Check sheet for the modelled part. Datum: model origin and axes. Units: mm. A direction names the side the tool comes from. Round coordinates to 2 decimals unless told otherwise and drop trailing zeros. Write each loop counter-clockwise with the first axis right and the second up, starting at its lowest first coordinate (ties: lowest second). Pieces come first, ordered by that corner, then holes. Notation, with made-up numbers: (14, -35) -> (37, -35) arc R14 cw to (37, -23) -> close; hole circle Ø10 at (5.5, -19.5). An arc over 180 degrees is marked (long way). Answer as a JSON object with one key per item and string values. Group by question number.
```python
from build123d import *

# Parameters (mm, degrees)
F3_DEPTH        = 70.001
F3_COPIES_COUNT = 20


# Not quite as in the source:
# - a feature of the source that left no trace in its solid (it failed there, or was rolled back) is left out
# - a pattern or mirror of a feature is missing from the dataset's text; its kind, count and spacing are read off the source's solid


with BuildPart() as f1:
    # F0 (on Front) → F1 (revolve)
    with BuildSketch(Plane.XZ):
        Polygon((35, -20), (35, 20), (-35, 20), (-35, -20), (-15, -20), (-15, -37.5), (-35, -37.5), (-35, -62.5), (35, -62.5), (35, -37.5), (15, -37.5), (15, -20), align=None)
    revolve(axis=Axis((-7.5, 0, -80), (-1, 0, 0)))

    # F2 (on face) → F3 (cut, through all)
    with BuildSketch(Plane.YZ.offset(35)):
        with BuildLine():
            ThreePointArc((-2.4875303205, 5.9552673354), (0.9594167449, 5.9859018055), (4.4048221019, 5.878363585))
            ThreePointArc((4.4048221019, 5.878363585), (5.5383005859, 6.1619770528), (6.3198858178, 7.0305014326))
            Line((6.3198858178, 7.0305014326), (12.0290632191, 19.2738718801))
            ThreePointArc((12.0290632191, 19.2738718801), (0, 20), (-12.0290632191, 19.2738718801))
            Line((-12.0290632191, 19.2738718801), (-7.1637078206, 8.8400835574))
            ThreePointArc((-7.1637078206, 8.8400835574), (-5.2573859952, 6.6977976646), (-2.4875303205, 5.9552673354))
        make_face()
    f3 = extrude(amount=-F3_DEPTH, mode=Mode.SUBTRACT)

    # F3_copies: F3 ×20 about axis
    f3_copies_axis = Axis((0, 0, -80), (1, 0, 0))
    for i in range(1, F3_COPIES_COUNT):
        add(f3.rotate(f3_copies_axis, i * 360 / F3_COPIES_COUNT), mode=Mode.SUBTRACT)


solid = f1.part
```
(1) Scan lines: line 1 along Y through (x, z) = (28.25, -80); line 2 along Z through (x, y) = (-27.5, 3); line 3 along Z through (x, y) = (-9.5, -87). Record each from-to range of solid material in increasing order.
(2) Release check for a two-part mould opening along Y. For faces 4 (the flat face through (0.49, 86.55, -41.75)), 5 (the cylindrical face through (0.49, 5.29, -166.72)), 6 (the cylindrical face through (-0.5, -45.4, 9.1)) record: pulls with the +Y half, pulls with the -Y half, needs draft (parallel to the pull), parting line crosses it, or undercut.
(3) Access from +Z, -Z, +X, -X, +Y, -Y to the whole of each face (thin tool, end or side, straight path). Record for faces 1 (the flat face through (0.49, -47.313, 0.661)), 2 (the flat face through (0.49, 69.92, -142.09)), 3 (the flat face through (0.49, -63.119, -9.508)).
(4) Section check C-C on x = 22.5. State how many separate pieces and enclosed holes the cut face has, then the cut area to 3 significant figures.
(5) Section check B-B on y = 0. Record the cut outline in (x, z).
(6) Go/stop test with flat-tipped pins: pin 1 Ø10 at (x, z) = (21, -53.5) entering from -Y; pin 2 Ø1 at (x, y) = (7, -59) entering from +Z; pin 3 Ø2 at (x, z) = (8, -0.5) entering from +Y. Record where each tip stops, or that it passes through.
(7) Section check A-A on z = -80. Record the cut outline in (x, y).
Data:
{
 "1": {"line 1": "y = -85.99 to -60, -42.5 to -17.5, 17.5 to 42.5, 60 to 85.99", "line 2": "z = -165.97 to -139.92, -122.39 to -97.24, -62.76 to -37.61, -20.08 to 5.94", "line 3": "z = -128.55 to -118.67, -100.6 to -85.69, -73.69 to -59.4, -41.33 to -31.45"},
 "2": {"face 4": "pulls with the +Y half", "face 5": "undercut", "face 6": "pulls with the -Y half"},
 "3": {"face 1": "+X, -X, -Y", "face 2": "+X, -X, +Y", "face 3": "+Z, +X, -X"},
 "4": {"separate pieces": "2", "enclosed holes": "2", "area": "19,900 mm²"},
 "5": {"outline": "(-35, -165.99) -> (35, -165.99) -> (35, -140) -> (15, -140) -> (15, -122.5) -> (35, -122.5) -> (35, -97.5) -> (-35, -97.5) -> (-35, -122.5) -> (-15, -122.5) -> (-15, -140) -> (-35, -140) -> close; (-35, -62.5) -> (35, -62.5) -> (35, -37.5) -> (15, -37.5) -> (15, -20) -> (35, -20) -> (35, 5.99) -> (-35, 5.99) -> (-35, -20) -> (-15, -20) -> (-15, -37.5) -> (-35, -37.5) -> close"},
 "6": {"pin 1": "stops at y = -84.46", "pin 2": "stops at z = -11.51", "pin 3": "stops at y = 47.28"},
 "7": {"outline": "(-35, -85.99) -> (35, -85.99) -> (35, -60) -> (15, -60) -> (15, -42.5) -> (35, -42.5) -> (35, -17.5) -> (-35, -17.5) -> (-35, -42.5) -> (-15, -42.5) -> (-15, -60) -> (-35, -60) -> close; (-35, 17.5) -> (35, 17.5) -> (35, 42.5) -> (15, 42.5) -> (15, 60) -> (35, 60) -> (35, 85.99) -> (-35, 85.99) -> (-35, 60) -> (-15, 60) -> (-15, 42.5) -> (-35, 42.5) -> close"}
}
